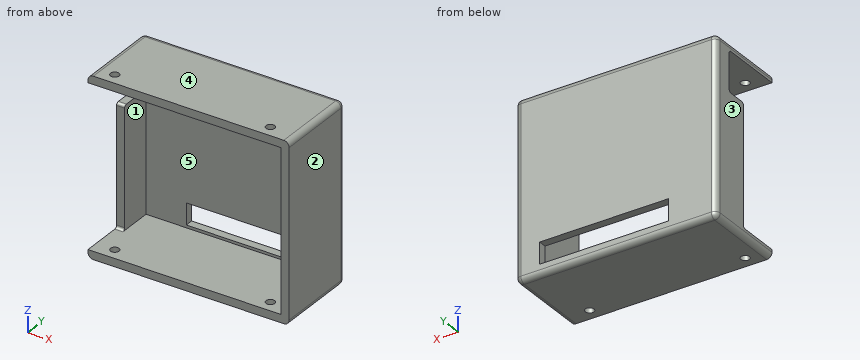
from build123d import *

# Parameters (mm, degrees)
SKETCH1_W               = 78
SKETCH1_H               = 66
SKETCH1_W_2             = 72
SKETCH1_H_2             = 60
BOSS_EXTRUDE1_DEPTH     = 28
SKETCH2_W               = 78
SKETCH2_H               = 66
SKETCH2_W_2             = 48
SKETCH2_H_2             = 8
BOSS_EXTRUDE2_DEPTH     = 3
SKETCH3_W               = 66
SKETCH3_H               = 31
CUT_EXTRUDE1_DEPTH      = 3
SKETCH5_W               = 45
SKETCH5_H               = 4
SKETCH5_W_2             = 15
BOSS_EXTRUDE4_DEPTH     = 3
SKETCH5_4_W             = 45
SKETCH5_4_H             = 8
BOSS_EXTRUDE5_DEPTH     = 3
FILLET1_R               = 1
FILLET2_R               = 2
SKETCH6_R               = 1.605618252
SKETCH6_R_2             = 1.6
CUT_EXTRUDE2_DEPTH      = 17
SKETCH6_3_R             = 1.605618252
SKETCH6_3_R_2           = 1.6
CUT_EXTRUDE4_DEPTH      = 103
CUT_EXTRUDE4_DEPTH_BACK = 17


with BuildPart() as part:
    # Sketch1 → Boss-Extrude1 (new body)
    with BuildSketch(Plane.XZ):
        with Locations((36, 28)):
            Rectangle(SKETCH1_W, SKETCH1_H)
        with Locations((36, 28)):
            Rectangle(SKETCH1_W_2, SKETCH1_H_2, mode=Mode.SUBTRACT)
    extrude(amount=-BOSS_EXTRUDE1_DEPTH)

    # Sketch2 → Boss-Extrude2 (add)
    with BuildSketch(Plane(origin=(0, 28, 0), x_dir=(1, 0, 0), z_dir=(0, 1, 0))):
        with Locations((36, -28)):
            Rectangle(SKETCH2_W, SKETCH2_H)
        with Locations((42, -3)):
            Rectangle(SKETCH2_W_2, SKETCH2_H_2, mode=Mode.SUBTRACT)
    extrude(amount=BOSS_EXTRUDE2_DEPTH)

    # Sketch3 → Cut-Extrude1 (cut)
    with BuildSketch(Plane.ZY.offset(3)):
        with Locations((28, 15.5)):
            Rectangle(SKETCH3_W, SKETCH3_H)
    extrude(amount=-CUT_EXTRUDE1_DEPTH, mode=Mode.SUBTRACT)

    # Sketch5 → Boss-Extrude4 (add)
    with BuildSketch(Plane.ZY):
        with Locations((20.5, 26)):
            Rectangle(SKETCH5_W, SKETCH5_H)
        with Locations((50.5, 26)):
            Rectangle(SKETCH5_W_2, SKETCH5_H)
    extrude(amount=-BOSS_EXTRUDE4_DEPTH)

    # Sketch5_4 → Boss-Extrude5 (add)
    with BuildSketch(Plane.ZY):
        with Locations((20.5, 20)):
            Rectangle(SKETCH5_4_W, SKETCH5_4_H)
    extrude(amount=-BOSS_EXTRUDE5_DEPTH)

    # Fillet1
    fillet1_edges = [part.edges().sort_by_distance(p)[0] for p in [
        (1.5, 24, 58),
        (1.5, 24, 43),
        (1.5, 16, 43),
        (1.5, 16, -2),
    ]]
    fillet(fillet1_edges, radius=FILLET1_R)

    # Fillet2
    fillet2_edges = [part.edges().sort_by_distance(p)[0] for p in [
        (75, 31, 28),
        (37.5, 31, 61),
        (37.5, 31, -5),
        (0, 15.5, -5),
        (0, 31, 28),
        (0, 15.5, 61),
        (75, 15.5, 61),
        (75, 15.5, -5),
    ]]
    fillet(fillet2_edges, radius=FILLET2_R)

    # Sketch6 → Cut-Extrude2 (cut)
    with BuildSketch(Plane(origin=(0, 0, 58), x_dir=(-1, 0, 0), z_dir=(0, 0, -1))):
        with Locations((-64.99455474, 4.498616562)):
            Circle(SKETCH6_R)
        with Locations((-7, 4.5)):
            Circle(SKETCH6_R_2)
    extrude(amount=-CUT_EXTRUDE2_DEPTH, mode=Mode.SUBTRACT)

    # Sketch6_3 → Cut-Extrude4 (cut, two sides)
    with BuildSketch(Plane(origin=(0, 0, 58), x_dir=(-1, 0, 0), z_dir=(0, 0, -1))) as cut_extrude4_sk:
        with Locations((-64.99455474, 4.498616562)):
            Circle(SKETCH6_3_R)
        with Locations((-7, 4.5)):
            Circle(SKETCH6_3_R_2)
    extrude(amount=CUT_EXTRUDE4_DEPTH, mode=Mode.SUBTRACT)
    extrude(cut_extrude4_sk.sketch, amount=-CUT_EXTRUDE4_DEPTH_BACK, mode=Mode.SUBTRACT)


solid = part.part
Model file for the job. Use its own axes, mm. Face numbers are marked on the shaded views. A direction names the side the tool comes from. Give positions to 0.01 mm unless a question says otherwise; leave off trailing zeros. Order: outer loops, then holes, each group sorted by start corner. A loop starts at its lowest first (then second) coordinate and runs counter-clockwise, first axis right, second up. Notation, with made-up numbers: M -25,-15 L 28,-15 A22 ccw 28,-6 Z; hole C -38,41.25 d11. An arc over 180 degrees is marked long. Put each result on its own line as item: value. Start each with the question number.
(1) Pull direction X, two halves, no side cores. Call the marked faces 1, 2 and 3: released by +X, released by -X, zero draft, split by the parting line, or undercut.
(2) Pin check, flat tips, straight feed: pin 1 Ø3 at (x, y) = (64.99, 4.5) entering from -Z; pin 2 Ø3.5 at (x, z) = (1.5, 52) entering from -Y; pin 3 Ø0.9 at (x, y) = (41.5, 30) entering from +Z; pin 4 Ø6 at (y, z) = (15, 49.5) entering from -X. Stop position of each tip, or through.
(3) Band-saw the part on C-C on z = 25.5. Give the cut face in (x, y), then the cut area to 3 significant figures.
(4) Band-saw the part on B-B on x = 40. Give the cut face in (y, z).
(5) Band-saw the part on A-A on x = 7. Give the cut face in (y, z), then the cut area to 3 significant figures.
(6) Drill centre lines: L1, parallel to Y at x = 7, z = -3; L2, parallel to Z at x = 54, y = 14.5; L3, parallel to X at y = 17, z = 14.5. Where is each one in solid material? Low to high. Write a range as [from, to].
(7) Band-saw the part on D-D on z = 53. Give the cut face in (x, y), then the cut area to 3 significant figures.
(8) Tool access for the marked faces 4 and 5: list every direction of +Z, -Z, +X, -X, +Y, -Y with a clear straight run to the whole face (end or side of a thin tool).
Results below:
1. face 1: undercut
1. face 2: released by +X
1. face 3: released by -X
2. pin 1: passes through
2. pin 2: stops at y = 24
2. pin 3: stops at z = 60.92
2. pin 4: stops at x = 72
3. outline: M 0,16 L 3,16 L 3,28 L 72,28 L 72,0 L 75,0 L 75,29 A2 ccw 73,31 L 2,31 A2 ccw 0,29 Z
3. area: 343 mm2
4. outline: M 0,-5 L 29,-5 A2 ccw 31,-3 L 31,-1 L 28,-1 L 28,-2 L 0,-2 Z; M 0,58 L 28,58 L 28,7 L 31,7 L 31,59 A2 ccw 29,61 L 0,61 Z
5. outline: M 0,-5 L 2.9,-5 L 2.9,-2 L 0,-2 Z; M 0,58 L 2.9,58 L 2.9,61 L 0,61 Z; M 6.1,-5 L 29,-5 A2 ccw 31,-3 L 31,59 A2 ccw 29,61 L 6.1,61 L 6.1,58 L 28,58 L 28,-2 L 6.1,-2 Z
5. area: 345 mm2
6. L1: y = [0, 2.9], [6.1, 31]
6. L2: z = [-5, -2], [58, 61]
6. L3: x = [0, 3], [72, 75]
7. outline: M 0,24 L 3,24 L 3,28 L 72,28 L 72,0 L 75,0 L 75,29 A2 ccw 73,31 L 2,31 A2 ccw 0,29 Z
7. area: 319 mm2
8. face 4: +Z, +X, -X, +Y, -Y
8. face 5: -Y
